Verification items for the finished model (mm, model axes). Give positions to 0.01 mm unless a question says otherwise; leave off trailing zeros. Write each loop counter-clockwise with the first axis right and the second up, starting at its lowest first coordinate (ties: lowest second). Pieces come first, ordered by that corner, then holes.
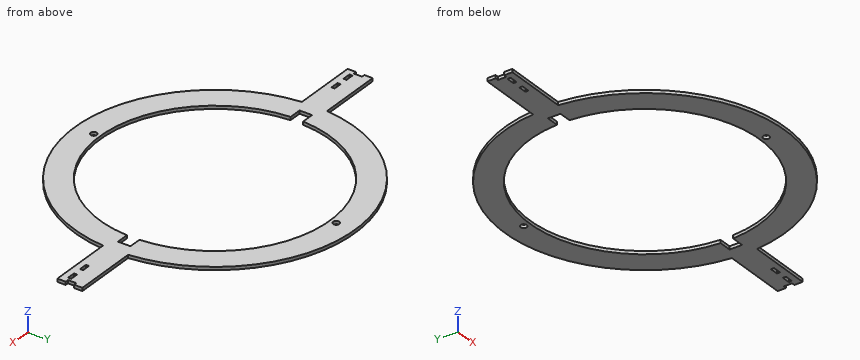
from build123d import *

# Parameters (mm, degrees)
SKETCH1_R           = 141.9733
SKETCH1_R_2         = 116.5733
BOSS_EXTRUDE1_DEPTH = 3.175
CUT_EXTRUDE1_START  = -3.175
SKETCH2_W           = 3.175
SKETCH2_H           = 8.466666666
CUT_EXTRUDE1_DEPTH  = 3.175
SKETCH3_R           = 3.175
CUT_EXTRUDE2_DEPTH  = 3.175
SKETCH4_W           = 8.466666667
SKETCH4_H           = 3.175
CUT_EXTRUDE3_DEPTH  = 3.175


with BuildPart() as part:
    # Sketch1 → Boss-Extrude1 (new body)
    # profile 1 of 3: a face of its own
    with BuildSketch(Plane.XY):
        with BuildLine():
            Line((-206.375, -12.7), (-141.404129759, -12.7))
            ThreePointArc((-141.404129759, -12.7), (-141.9733, 0), (-141.404129759, 12.7))
            Line((-141.404129759, 12.7), (-206.375, 12.7))
            Line((-206.375, 12.7), (-206.375, -12.7))
        make_face()
    # profile 2 of 3: a face of its own
    with BuildSketch(Plane.XY):
        Circle(SKETCH1_R)
        Circle(SKETCH1_R_2, mode=Mode.SUBTRACT)
    # profile 3 of 3: a face of its own
    with BuildSketch(Plane.XY):
        with BuildLine():
            ThreePointArc((141.9733, 0), (141.830936062, -6.356373863), (141.404129759, -12.7))
            Line((141.404129759, -12.7), (206.375, -12.7))
            Line((206.375, -12.7), (206.375, 12.7))
            Line((206.375, 12.7), (141.404129759, 12.7))
            ThreePointArc((141.404129759, 12.7), (141.830936062, 6.356373863), (141.9733, 0))
        make_face()
    extrude(amount=BOSS_EXTRUDE1_DEPTH)

    # Sketch2 → Cut-Extrude1 (cut)
    with BuildSketch(Plane.XY.offset(3.175).offset(CUT_EXTRUDE1_START)):
        with Locations((-204.7875, 0)):
            Rectangle(SKETCH2_W, SKETCH2_H)
        with BuildLine():
            Line((-116.400222392, 6.35), (-129.100222392, 6.35))
            Line((-129.100222392, 6.35), (-129.100222392, -6.35))
            Line((-129.100222392, -6.35), (-116.400222392, -6.35))
            ThreePointArc((-116.400222392, -6.35), (-116.5733, 0), (-116.400222392, 6.35))
        make_face()
    cut_extrude1 = extrude(amount=CUT_EXTRUDE1_DEPTH, mode=Mode.SUBTRACT)

    # Mirror1: Cut-Extrude1 across plane
    add(cut_extrude1.mirror(Plane(origin=(0, 0, 0), x_dir=(0, 0, 1), z_dir=(1, 0, 0))), mode=Mode.SUBTRACT)

    # Sketch3 → Cut-Extrude2 (cut)
    with BuildSketch(Plane.XY.offset(3.175)):
        with Locations((0, 122.936)):
            Circle(SKETCH3_R)
    cut_extrude2 = extrude(amount=-CUT_EXTRUDE2_DEPTH, mode=Mode.SUBTRACT)

    # Mirror2: Cut-Extrude2 across plane
    add(cut_extrude2.mirror(Plane.ZX), mode=Mode.SUBTRACT)

    # Sketch4 → Cut-Extrude3 (cut)
    with BuildSketch(Plane.XY.offset(3.175)):
        with Locations((195.791666667, -4.7625)):
            Rectangle(SKETCH4_W, SKETCH4_H)
        with Locations((178.858333334, -4.7625)):
            Rectangle(SKETCH4_W, SKETCH4_H)
    cut_extrude3 = extrude(amount=-CUT_EXTRUDE3_DEPTH, mode=Mode.SUBTRACT)

    # Mirror3: Cut-Extrude3 across plane
    add(cut_extrude3.mirror(Plane(origin=(0, 0, 0), x_dir=(0, 0, 1), z_dir=(1, 0, 0))), mode=Mode.SUBTRACT)


solid = part.part
Item 1: Sectioned sample at A-A on x = 107.5. Record the cut outline in (y, z) (3 decimals).
Answer key:
outline: (-92.737, 0) - (-45.09, 0) - (-45.09, 3.175) - (-92.737, 3.175) - close; (45.09, 0) - (92.737, 0) - (92.737, 3.175) - (45.09, 3.175) - close
Item 2: Sectioned sample at C-C on z = 0.5. State how many separate pieces and enclosed holes the cut face has, then the cut area to 3 significant figures.
Answer key:
separate pieces: 1
enclosed holes: 7
area: 23,400 mm2
Item 3: Sectioned sample at B-B on y = -57. Record the cut outline in (x, z) (3 decimals), then the cut area to 3 significant figures.
Answer key:
outline: (-130.029, 0) - (-101.687, 0) - (-101.687, 3.175) - (-130.029, 3.175) - close; (101.687, 0) - (130.029, 0) - (130.029, 3.175) - (101.687, 3.175) - close
area: 180 mm2
Item 4: Depth check by flat-ended pin: pin 1 (1 mm diameter, centred on x = 172.5, z = 2, fed in from -Y); pin 2 (1.6 mm diameter, centred on x = 179, z = 2.5, fed in from +Y); pin 3 (1 mm diameter, centred on y = -21, z = 2.5, fed in from +X); pin 4 (4 mm diameter, centred on x = 0, y = -122.936, fed in from +Z). Enter the tip coordinate at first touch or a pass-through.
Answer key:
pin 1: stops at y = -12.7
pin 2: stops at y = 12.7
pin 3: stops at x = 140.49
pin 4: passes through
Item 5: Scan lines: line 1 along X through (y, z) = (-6.5, 2.9) (3 decimals); line 2 along X through (y, z) = (-97.5, 0.6); line 3 along Y through (x, z) = (16.5, 2.1). Record each from-to range of solid material in increasing order.
Answer key:
line 1: x = -206.375 to -116.392, 116.392 to 206.375
line 2: x = -103.2 to -63.9, 63.9 to 103.2
line 3: y = -141.01 to -115.4, 115.4 to 141.01
